Can you work these out from the model? Positions are in its coordinate system, mm. Face numbers are marked on the shaded views. A direction names the side the tool comes from. Coordinates: 2 decimals unless noted, no trailing zeros. Loops run counter-clockwise (first coordinate to the right, second up) from the corner with the lowest first, then second, coordinate; pieces in that order, holes last.
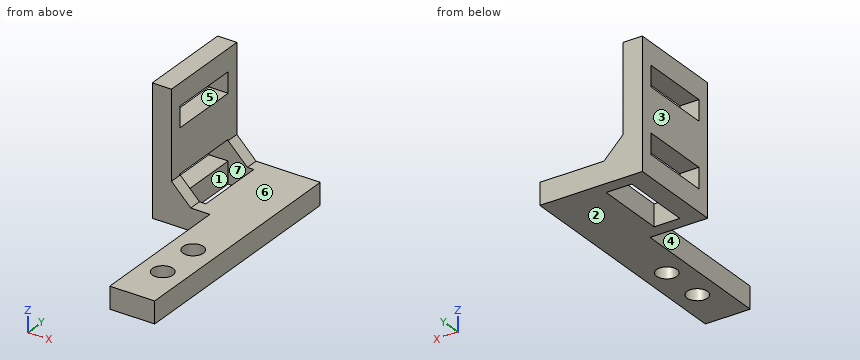
Autodesk Inventor part; units mm, degrees
ref_plane "YZ Plane" through (0, 0, 0) normal (1, 0, 0) x (0, 1, 0)
ref_plane "XZ Plane" through (0, 0, 0) normal (0, 1, 0) x (-1, 0, 0)
ref_plane "XY Plane" through (0, 0, 0) normal (0, 0, 1) x (1, 0, 0)
sketch "Sketch1" plane through (0, 0, 0) normal (0, 0, 1) x (1, 0, 0)
  line L0 (0, 0) -> (7, 0)
  line L1 (7, 0) -> (7, 38)
  line L2 (7, 38) -> (0, 38)
  line L3 (0, 38) -> (0, 0)
  circle A0 centre (3.5, 7) radius 1.6
  circle A1 centre (3.5, 14) radius 1.6
  line L4 (0, 38) -> (-9, 38)
  line L5 (-9, 38) -> (-9, 23)
  line L6 (-9, 23) -> (0, 23)
  line L7 (0, 23) -> (0, 38)
  point P0 (3.5, 0)
  dimension "d0" = 7
  dimension "d1" = 38
  dimension "d2" = 3.2
  dimension "d3" = 3.2
  dimension "d4" = 7
  dimension "d5" = 7
  dimension "d7" = 15
  dimension "d8" = 16
extrude "Extrusion1" add sketch "Sketch1" along normal blind 3.4
sketch "Sketch2" plane through (-9, 23, 0) normal (-1, 0, 0) x (0, 0, 1)
  line L0 (0, 15) -> (0, 0)
  line L1 (0, 0) -> (3.4, 0)
  line L2 (3.4, 15) -> (3.4, 0)
  line L3 (0, 15) -> (3.4, 15)
  line L4 (0, 15) -> (20, 15)
  line L5 (20, 15) -> (20, 0)
  line L6 (20, 0) -> (0, 0)
  line L7 (0, 0) -> (0, 15)
  line L8 (3.4, 13) -> (6.6, 13)
  line L9 (6.6, 13) -> (6.6, 2)
  line L10 (6.6, 2) -> (3.4, 2)
  line L11 (3.4, 2) -> (3.4, 13)
  line L12 (13.4, 13) -> (16.6, 13)
  line L13 (16.6, 13) -> (16.6, 2)
  line L14 (16.6, 2) -> (13.4, 2)
  line L15 (13.4, 2) -> (13.4, 13)
  point P0 (0, -23)
  dimension "d11" = 20
  dimension "d12" = 2
  dimension "d13" = 2
  dimension "d14" = 3.2
  dimension "d15" = 3.4
  dimension "d16" = 6.8
  dimension "d17" = 3.2
extrude "Extrusion2" add sketch "Sketch2" against normal blind 3 contours L4 L5 L6 L2 L10 L9 L8
chamfer "Chamfer1" distance 3 angle 45 2 edges at (-6, 37, 3.4) (-6, 24, 3.4)
sketch "Sketch3" plane through (0, 0, 3.4) normal (0, 0, 1) x (1, 0, 0)
  line L0 (-9, 25) -> (-6, 25)
  line L1 (-6, 36) -> (-2, 36)
  line L2 (-2, 36) -> (-2, 25)
  line L3 (-2, 25) -> (-6, 25)
  line L4 (-6, 25) -> (-6, 36)
  dimension "d20" = 4
extrude "Extrusion3" cut sketch "Sketch3" against normal blind 4
equation "\"d13\" = d12"
equation "\"d17\" = d14"
properties part number "switch bracket v5"
Item 1: I'm going to push flat-ended pins straight in: P1, Ø1.5, axis at x = -3.5, y = 25, coming from the +Z side; P2, Ø3, axis at x = -7.5, z = 12.5, coming from the -Y side; P3, Ø1.5, axis at x = 4, y = 4.5, coming from the -Z side; P4, Ø4, axis at y = 32, z = 14.5, coming from the +X side. Where does each tip first touch, or does it pass through?
Results are:
P1: stops at z = 4.65
P2: stops at y = 23
P3: stops at z = 0
P4: stops at x = -6
Item 2: Suppose I cut it at D-D, the plane x = -2.5. Please give me the cut outline in (y, z), plus the area to 3 significant figures.
Results are:
outline: (23, 0) - (25, 0) - (25, 3.4) - (23, 3.4) - close; (36, 0) - (38, 0) - (38, 3.4) - (36, 3.4) - close
area: 13.6 mm2
Item 3: Suppose I cut it at A-A, the plane y = 28.5. Please give me the cut outline in (x, z).
Results are:
outline: (-9, 0) - (-6, 0) - (-6, 3.4) - (-9, 3.4) - close; (-9, 6.6) - (-6, 6.6) - (-6, 13.4) - (-9, 13.4) - close; (-9, 16.6) - (-6, 16.6) - (-6, 20) - (-9, 20) - close; (-2, 0) - (7, 0) - (7, 3.4) - (-2, 3.4) - close
Item 4: Suppose I cut it at B-B, the plane x = 3.5. Please give me the cut outline in (y, z).
Results are:
outline: (0, 0) - (5.4, 0) - (5.4, 3.4) - (0, 3.4) - close; (8.6, 0) - (12.4, 0) - (12.4, 3.4) - (8.6, 3.4) - close; (15.6, 0) - (38, 0) - (38, 3.4) - (15.6, 3.4) - close
Item 5: I need wall thicknesses on line 1 along Y through (x, z) = (3.5, 1.65); line 2 along Y through (x, z) = (-8, 16.5); line 3 along X through (y, z) = (25.5, 7.75). Which ranges of each line are inside material? Lowest first, please.
Results are:
line 1: y = 0 to 5.4, 8.6 to 12.4, 15.6 to 38
line 2: y = 23 to 25, 36 to 38
line 3: x = -9 to -6
Item 6: We'd pull the mould along X, two halves only. Please class the marked faces 1, 2 and 3: +X half, -X half, draft (parallel to the pull), parting line (faces both ways), or undercut.
Results are:
face 1: undercut
face 2: draft
face 3: -X half
Item 7: On a 3-axis mill with a long thin cutter (end or side, diameter ignored), from which of +Z, -Z, +X, -X, +Y, -Y can I reach the whole of each face in a straight line? I mean the marked faces 4, 5, 6 and 7. Say none if no direction works.
Results are:
face 4: +Z, -Z, -X, -Y
face 5: +X, -X
face 6: +Z, +X, +Y, -Y
face 7: none
Item 8: Suppose I cut it at C-C, the plane z = 5.75. Please give me the cut outline in (x, y).
Results are:
outline: (-9, 23) - (-5.35, 23) - (-5.35, 25) - (-9, 25) - close; (-9, 36) - (-5.35, 36) - (-5.35, 38) - (-9, 38) - close
